```python
from build123d import *

# Parameters (mm, degrees)
BOSS_EXTRUDE1_DEPTH = 19.05
SKETCH2_W           = 43.434
SKETCH2_H           = 13.97
MOTOR_HOLE_DEPTH    = 19.05
SKETCH3_W           = 6.35
SKETCH3_H           = 12.7
CUT_EXTRUDE2_DEPTH  = 36.941
SKETCH5_W           = 6.35
SKETCH5_H           = 13.97
SKETCH5_H_2         = 6.35
CUT_EXTRUDE6_DEPTH  = 36.941
SKETCH7_W           = 50.257507562
SKETCH7_H           = 159.787423729
CUT_EXTRUDE7_DEPTH  = 20.05


with BuildPart() as part:
    # Sketch1 → Boss-Extrude1 (new body)
    with BuildSketch(Plane(origin=(0, 0, 0), x_dir=(1, 0, 0), z_dir=(0, 1, 0))):
        Polygon((-10.033, 66.167), (-11.6205, 66.167), (-11.6205, 76.835), (-17.9705, 76.835), (-17.9705, -78.867), (-11.6205, -78.867), (-11.6205, -66.167), (11.6205, -66.167), (11.6205, -78.867), (17.9705, -78.867), (17.9705, 76.835), (11.6205, 76.835), (11.6205, 66.167), (10.033, 66.167), (10.033, 59.817), (11.6205, 59.817), (11.6205, -59.817), (-11.6205, -59.817), (-11.6205, 59.817), (-10.033, 59.817), align=None)
    extrude(amount=BOSS_EXTRUDE1_DEPTH)

    # Sketch2 → Motor Hole (cut)
    with BuildSketch(Plane.ZY.offset(17.9705)):
        with Locations((29.972, 12.065)):
            Rectangle(SKETCH2_W, SKETCH2_H)
    extrude(amount=-MOTOR_HOLE_DEPTH, mode=Mode.SUBTRACT)

    # Sketch3 → Cut-Extrude2 (cut, through all)
    with BuildSketch(Plane.ZY.offset(17.9705)):
        with Locations((-73.66, 6.35)):
            Rectangle(SKETCH3_W, SKETCH3_H)
    extrude(amount=-CUT_EXTRUDE2_DEPTH, mode=Mode.SUBTRACT)

    # Sketch5 → Cut-Extrude6 (cut, through all)
    with BuildSketch(Plane.ZY.offset(17.9705)):
        with Locations((62.992, 12.065)):
            Rectangle(SKETCH5_W, SKETCH5_H)
        with Locations((-62.992, 9.525)):
            Rectangle(SKETCH5_W, SKETCH5_H_2)
    extrude(amount=-CUT_EXTRUDE6_DEPTH, mode=Mode.SUBTRACT)

    # Sketch7 → Cut-Extrude7 (cut, through all)
    with BuildSketch(Plane(origin=(0, 0, 0), x_dir=(1, 0, 0), z_dir=(0, 1, 0))):
        with Locations((13.508253781, 1.026711865)):
            Rectangle(SKETCH7_W, SKETCH7_H)
    extrude(amount=CUT_EXTRUDE7_DEPTH, mode=Mode.SUBTRACT)


solid = part.part
```
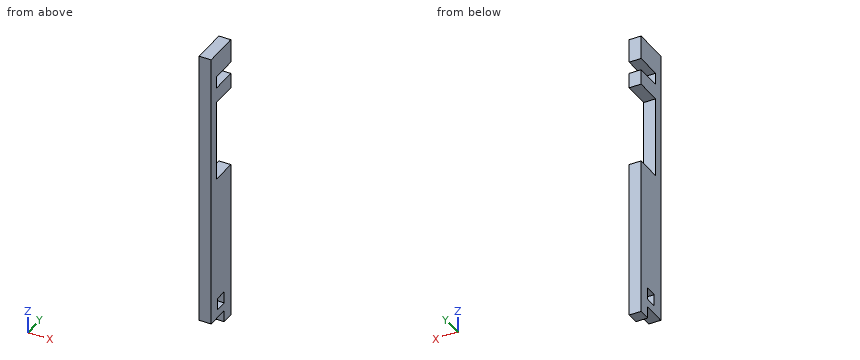
Can you work these out from the model? Positions are in its coordinate system, mm. Give positions to 0.01 mm unless a question says otherwise; leave off trailing zeros. Loops run counter-clockwise (first coordinate to the right, second up) from the corner with the lowest first, then second, coordinate; pieces in that order, holes last. Notation, with made-up numbers: M -34,1 L -6,1 A19 cw -6,8 Z; hole C -24,-23 d8. An arc over 180 degrees is marked long. Answer in a Markdown table with one row per item.
1. Suppose I cut it at D-D on z = 22. Write out the boundary of the cut face in (x, y), plus the area to 3 significant figures.
Taken from the geometry:
| item | result |
|---|---|
| outline | M -17.97,0 L -11.62,0 L -11.62,5.08 L -17.97,5.08 Z |
| area | 32.3 mm² |
2. Suppose I cut it at C-C on x = -14.5. Write out the boundary of the cut face in (y, z) (3 decimals).
Taken from the geometry:
| item | result |
|---|---|
| outline | M 0,-70.485 L 12.7,-70.485 L 12.7,-76.835 L 19.05,-76.835 L 19.05,8.255 L 5.08,8.255 L 5.08,51.689 L 19.05,51.689 L 19.05,59.817 L 5.08,59.817 L 5.08,66.167 L 19.05,66.167 L 19.05,78.867 L 0,78.867 Z; hole M 6.35,-66.167 L 12.7,-66.167 L 12.7,-59.817 L 6.35,-59.817 Z |
3. If I drill on line 1 along Z through (x, y) = (-15, 13.75) (3 decimals); line 2 along Z through (x, y) = (-13, 8.5) (3 decimals); line 3 along Y through (x, z) = (-16.25, 30.5), over which ranges is the centre line in solid material (lowest first)?
Taken from the geometry:
| item | result |
|---|---|
| line 1 | z = -76.835 to 8.255, 51.689 to 59.817, 66.167 to 78.867 |
| line 2 | z = -70.485 to -66.167, -59.817 to 8.255, 51.689 to 59.817, 66.167 to 78.867 |
| line 3 | y = 0 to 5.08 |
4. For pin 1 Ø3 at (x, y) = (-14, 9.5) entering from -Z (3 decimals); pin 2 Ø6 at (y, z) = (8.5, 21) entering from -X; pin 3 Ø1.9 at (x, z) = (-14, 62) entering from +Y, each with a flat end and sliding along its axis, tell me the tip position at first contact or that it passes through.
Taken from the geometry:
| item | result |
|---|---|
| pin 1 | stops at z = -70.485 |
| pin 2 | passes through |
| pin 3 | stops at y = 5.08 |
5. Suppose I cut it at A-A on y = 17.5. Write out the boundary of the cut face in (x, z) (1 decimal), plus the area to 3 significant figures.
Taken from the geometry:
| item | result |
|---|---|
| outline | M -18,-76.8 L -11.6,-76.8 L -11.6,8.3 L -18,8.3 Z; M -18,51.7 L -11.6,51.7 L -11.6,59.8 L -18,59.8 Z; M -18,66.2 L -11.6,66.2 L -11.6,78.9 L -18,78.9 Z |
| area | 673 mm² |
6. Suppose I cut it at B-B on y = 9.5. Write out the boundary of the cut face in (x, z) (1 decimal).
Taken from the geometry:
| item | result |
|---|---|
| outline | M -18,-70.5 L -11.6,-70.5 L -11.6,-66.2 L -18,-66.2 Z; M -18,-59.8 L -11.6,-59.8 L -11.6,8.3 L -18,8.3 Z; M -18,51.7 L -11.6,51.7 L -11.6,59.8 L -18,59.8 Z; M -18,66.2 L -11.6,66.2 L -11.6,78.9 L -18,78.9 Z |
